Input: part model. Units: mm. Frame: model coordinates. Coordinates: 2 decimals unless noted, no trailing zeros. Write each loop counter-clockwise with the first axis right and the second up, starting at its lowest first coordinate (ties: lowest second). Pieces come first, ordered by that corner, then holes. Notation, with made-up numbers: M 46.25,69 L 75.25,69 A27 ccw 75.25,97 Z; hole C 53,71 d5. An arc over 180 degrees is marked long. Answer as a JSON object with one key per item and string values. Group by question number.
from build123d import *

# Parameters (mm, degrees)
SKETCH1_W                = 80
SKETCH1_H                = 50
BOSS_EXTRUDE1_DEPTH      = 8
FILLET1_R                = 2
M5_CLEARANCE_HOLE1_D     = 5.3
M5_CLEARANCE_HOLE1_DEPTH = 8
M5_CLEARANCE_HOLE1_TIP   = 1.59228064


with BuildPart() as part:
    # Sketch1 → Boss-Extrude1 (new body)
    with BuildSketch(Plane(origin=(0, 0, 0), x_dir=(1, 0, 0), z_dir=(0, 1, 0))):
        Rectangle(SKETCH1_W, SKETCH1_H)
    extrude(amount=BOSS_EXTRUDE1_DEPTH)

    # Fillet1
    fillet1_edges = [part.edges().sort_by_distance(p)[0] for p in [
        (-40, 4, -25),
        (40, 4, -25),
        (40, 4, 25),
        (-40, 4, 25),
    ]]
    fillet(fillet1_edges, radius=FILLET1_R)

    # M5 Clearance Hole1
    with Locations(Plane(origin=(0, 8, 0), x_dir=(1, 0, 0), z_dir=(0, 1, 0))):
        with Locations((-30, 15), (-16, 15), (-16, -15), (-30, -15), (30, -15), (16, -15), (16, 15), (30, 15)):
            Hole(M5_CLEARANCE_HOLE1_D / 2, depth=M5_CLEARANCE_HOLE1_DEPTH)
            with Locations((0, 0, -(M5_CLEARANCE_HOLE1_DEPTH + M5_CLEARANCE_HOLE1_TIP / 2))):  # 118° drill point
                Cone(0, M5_CLEARANCE_HOLE1_D / 2, M5_CLEARANCE_HOLE1_TIP, mode=Mode.SUBTRACT)


solid = part.part
Q1. Section B-B, the plane x = -30. Return the cut outline in (y, z), and give its area (3 significant figures).
Q2. Line query: line 1 (X direction, y = 4.5, z = -15); line 2 (Z direction, x = -30, y = 3.5); line 3 (Z direction, x = -28, y = 4.25). Output: solid intervals per line, ascending. Write a range as from..to.
Q3. Section D-D, the plane x = 31. Return the cut outline in (y, z), and give its area (3 significant figures).
Q4. Draft query along Z for faces 1 (the cylindrical face through (32.647, 3.944, -15.117)), 2 (the flat face through (-1, 0, 0)), 3 (the cylindrical face through (39.43, 4.06, -24.4)). Return one class per face: released by +Z, released by -Z, zero draft, split by the parting line, or undercut.
Q5. Section A-A, the plane y = 2.25. State how many separate pieces and enclosed holes the cut face has, and give its area (3 significant figures).
Q6. Section C-C, the plane z = 15. Return the cut outline in (x, y), and give its area (3 significant figures).
Q7. Pin query (flat end, axial travel): pin 1 Ø4 at (x, z) = (-16, -15) entering from -Y. Return the tip coordinate at first contact, or that it passes through.
Filled in:
{
 "1": {"outline": "M 0,-25 L 8,-25 L 8,-17.65 L 0,-17.65 Z; M 0,-12.35 L 8,-12.35 L 8,12.35 L 0,12.35 Z; M 0,17.65 L 8,17.65 L 8,25 L 0,25 Z", "area": "315 mm^2"},
 "2": {"line 1": "-40..-32.65, -27.35..-18.65, -13.35..13.35, 18.65..27.35, 32.65..40", "line 2": "-25..-17.65, -12.35..12.35, 17.65..25", "line 3": "-25..-16.74, -13.26..13.26, 16.74..25"},
 "3": {"outline": "M 0,-25 L 8,-25 L 8,-17.45 L 0,-17.45 Z; M 0,-12.55 L 8,-12.55 L 8,12.55 L 0,12.55 Z; M 0,17.45 L 8,17.45 L 8,25 L 0,25 Z", "area": "321 mm^2"},
 "4": {"face 1": "undercut", "face 2": "zero draft", "face 3": "released by -Z"},
 "5": {"separate pieces": "1", "enclosed holes": "8", "area": "3,820 mm^2"},
 "6": {"outline": "M -40,0 L -32.65,0 L -32.65,8 L -40,8 Z; M -27.35,0 L -18.65,0 L -18.65,8 L -27.35,8 Z; M -13.35,0 L 13.35,0 L 13.35,8 L -13.35,8 Z; M 18.65,0 L 27.35,0 L 27.35,8 L 18.65,8 Z; M 32.65,0 L 40,0 L 40,8 L 32.65,8 Z", "area": "470 mm^2"},
 "7": {"pin 1": "through"}
}
